The listing builds one solid part. Answer for the finished solid, in the listing's coordinates (mm). A direction names the side the tool comes from. Coordinates: 2 decimals unless noted, no trailing zeros. Write each loop counter-clockwise with the first axis right and the second up, starting at its lowest first coordinate (ties: lowest second). Pieces come first, ordered by that corner, then holes.
Autodesk Inventor part; units mm, degrees
ref_plane "YZ Plane" through (0, 0, 0) normal (1, 0, 0) x (0, 1, 0)
ref_plane "XZ Plane" through (0, 0, 0) normal (0, 1, 0) x (-1, 0, 0)
ref_plane "XY Plane" through (0, 0, 0) normal (0, 0, 1) x (1, 0, 0)
sketch "Esquisse1" plane through (0, 0, 0) normal (0, 0, 1) x (1, 0, 0)
  line L0 (0, 0) -> (-10, 0)
  line L1 (-10, 0) -> (-10, 30)
  line L2 (-10, 30) -> (0, 30)
  line L3 (0, 0) -> (-5, 0)
  line L4 (-5, 0) -> (-5, 5)
  line L5 (-5, 5) -> (0, 5)
  line L6 (0, 5) -> (0, 0)
  line L7 (0, 4) -> (-3, 4)
  line L8 (-3, 4) -> (-3, 1)
  line L9 (-3, 1) -> (0, 1)
  line L10 (0, 1) -> (0, 4)
  line L11 (-1.5, 5) -> (-1.5, 20)
  line L12 (-1.5, 20) -> (0, 20)
  line L13 (0, 30) -> (0, 20)
  line L14 (0, 5) -> (0, 0)
  line L15 (0, 29) -> (-3, 29)
  line L16 (-3, 29) -> (-3, 26)
  line L17 (-3, 26) -> (0, 26)
  line L18 (0, 26) -> (0, 29)
  line L19 (0, 25) -> (-5, 25)
  line L20 (-5, 25) -> (-5, 30)
  line L21 (-5, 25) -> (-7.5, 25)
  line L22 (-7.5, 25) -> (-7.5, 27.5)
  line L23 (-7.5, 27.5) -> (-5, 27.5)
  line L24 (-5, 27.5) -> (-5, 25)
  line L25 (-5, 0) -> (-7.5, 0)
  line L26 (-5, 2.5) -> (-5, 0)
  line L27 (-5, 5) -> (-7.5, 5)
  line L28 (-7.5, 5) -> (-7.5, 2.5)
  line L29 (-7.5, 2.5) -> (-5, 2.5)
  line L30 (-5, 2.5) -> (-5, 5)
  line L31 (-3, 26) -> (0, 26)
  line L32 (0, 26) -> (0, 29)
  line L33 (0, 29) -> (-3, 29)
  line L34 (-3, 29) -> (-3, 26)
  line L35 (-3, 1) -> (0, 1)
  line L36 (0, 1) -> (0, 4)
  line L37 (0, 4) -> (-3, 4)
  line L38 (-3, 4) -> (-3, 1)
  dimension "d0" = 10
  dimension "d1" = 30
  dimension "d2" = 5
  dimension "d3" = 5
  dimension "d4" = 3
  dimension "d5" = 3
  dimension "d6" = 1
  dimension "d7" = 15
  dimension "d9" = 3
  dimension "d10" = 3
  dimension "d11" = 1
  dimension "d12" = 5
  dimension "d13" = 5
  dimension "d14" = 2.5
  dimension "d15" = 2.5
  dimension "d20" = 2.5
  dimension "d21" = 2.5
extrude "Extrusion1" add sketch "Esquisse1" along normal blind 41.5 contours L0 L4 L5 L6 L7 L8 L9 | L9 L8 L7 L6 | L2 L13 L15 L16 L17 L19 L20 | L13 L17 L16 L15
extrude "Extrusion2" add sketch "Esquisse1" along normal blind 35 contours L29 L28 L27 L4 | L20 L21 L22 L23
extrude "Extrusion4" add sketch "Esquisse1" along normal blind 2 contours L0 L1 L2 L20 L23 L22 L21 L19 L13 L12 L11 L5 L27 L28 L29 L4
fillet "Congé1" radius 5 2 edges at (-10, 0, 1) (-10, 30, 1)
sketch "Esquisse3" plane through (0, 0, 0) normal (0, 0, -1) x (-1, 0, 0)
  circle A0 centre (7, 9) radius 0.7
  circle A1 centre (7, 21) radius 0.7
  line L0 (0, 0) -> (0, 5)
  line L1 (0, 20) -> (0, 30)
  line L2 (5, 0) -> (0, 0)
  dimension "d29" = 1.4
  dimension "d30" = 1.4
  dimension "d31" = 12
  dimension "d32" = 7
  dimension "d33" = 7
  dimension "d34" = 9
extrude "Extrusion5" cut sketch "Esquisse3" against normal through all
fillet "Congé2" radius 2 2 edges at (-3.75, 25, 2) (-4.5, 5, 2)
sketch "Esquisse8" plane through (0, 0, 41.5) normal (0, 0, 1) x (1, 0, 0)
  line L0 (0, 0) -> (0, 5)
  line L1 (0, 5) -> (-5, 5)
  line L2 (-5, 5) -> (-5, 0)
  line L3 (-5, 0) -> (0, 0)
  line L4 (0, 30) -> (-5, 30)
  line L5 (-5, 30) -> (-5, 25)
  line L6 (-5, 25) -> (0, 25)
  line L7 (0, 25) -> (0, 30)
  circle A0 centre (-2.5, 2.5) radius 2.4
  circle A1 centre (-2.5, 27.5) radius 2.4
  dimension "d42" = 4.8
  dimension "d43" = 2.5
  dimension "d44" = 2.5
  dimension "d45" = 4.8
  dimension "d48" = 2.5
  dimension "d49" = 2.5
extrude "Extrusion8" cut sketch "Esquisse8" against normal blind 6.5
sketch "Esquisse9" plane through (-2.5, 2.5, 41.5) normal (0, 0, 1) x (1, 0, 0)
  circle A0 centre (0, 0) radius 2.4
  circle A1 centre (0, 25) radius 2.4
  line L0 (0, 0) -> (3.9146, 0)
  circle A2 centre (1, 0) radius 1.4
  circle A3 centre (0, 0) radius 2.4
  line L1 (0, 25) -> (4.0517, 25)
  circle A4 centre (1, 25) radius 1.4
  point P0 (2.5, -2.5)
  dimension "d52" = 2.8
  dimension "d53" = 2.8
extrude "Extrusion9" cut sketch "Esquisse9" against normal blind 1.5
properties part number "blue_part-july21" material "Plastique ABS"
1. Section B-B on y = 9 is taken. Give the vertices of the cut face in (x, z).
Results found:
outline: (-10, 0) - (-7.7, 0) - (-7.7, 2) - (-10, 2) - close; (-6.3, 0) - (-1.5, 0) - (-1.5, 2) - (-6.3, 2) - close
2. For a pull along X with two mould halves and no side action, classify faces 1 (the cylindrical face through (-2.81, 4.88, 37.53)), 2 (the cylindrical face through (-6.909, 21.694, 0.986)), 3 (the flat face through (-3, 30, 17)) as pulls with the +X half, pulls with the -X half, needs draft (parallel to the pull), parting line crosses it, or undercut.
Results found:
face 1: parting line crosses it
face 2: undercut
face 3: needs draft
3. Section C-C on x = -1 is taken. Give the vertices of the cut face in (y, z), then the cut area to 3 significant figures.
Results found:
outline: (0, 0) - (5, 0) - (5, 35) - (4.37, 35) - (4.37, 40) - (3.81, 40) - (3.81, 41.5) - (1.19, 41.5) - (1.19, 40) - (0.63, 40) - (0.63, 35) - (0, 35) - close; (20, 0) - (30, 0) - (30, 35) - (29.37, 35) - (29.37, 40) - (28.81, 40) - (28.81, 41.5) - (26.19, 41.5) - (26.19, 40) - (25.63, 40) - (25.63, 35) - (25, 35) - (25, 4) arc R2 cw to (23, 2) - (20, 2) - close
area: 406 mm2
4. Flat-ended cylindrical pins translate along their axes: P1, Ø1.8, axis at x = -7, y = 9, coming from the +Z side; P2, Ø1.1, axis at x = -7, y = 21, coming from the -Z side; P3, Ø3.5, axis at y = 3.5, z = 18.5, coming from the -X side; P4, Ø3, axis at y = 12.5, z = 2, coming from the +X side. Find the tip coordinate at first contact, or state that the pin passes through.
Results found:
P1: stops at z = 2
P2: passes through
P3: stops at x = -7.5
P4: stops at x = -1.5
5. Find the intervals of material crossed by L1, parallel to Y at x = -7, z = 1.4; L2, parallel to Y at x = -6.5, z = 11; L3, parallel to Y at x = -3, z = 30, in increasing order.
Results found:
L1: y = 0.42 to 8.3, 9.7 to 20.3, 21.7 to 29.58
L2: y = 2.5 to 5, 25 to 27.5
L3: y = 0 to 5, 25 to 30
6. Section A-A on z = 17.5 is taken. Give the vertices of the cut face in (x, y), then the cut area to 3 significant figures.
Results found:
outline: (-7.5, 2.5) - (-5, 2.5) - (-5, 0) - (0, 0) - (0, 5) - (-7.5, 5) - close; (-7.5, 25) - (0, 25) - (0, 30) - (-5, 30) - (-5, 27.5) - (-7.5, 27.5) - close
area: 62.5 mm2
7. A tool of negligible diameter and unlimited length cuts with its end or side. For faces 4 (the cylindrical face through (-4.46, 5.57, 2.6)), 5 (the flat face through (-7.5, 26, 18)), 6 (the cylindrical face through (-1.803, 1.133, 40.76)), 7 (the flat face through (-6, 2.5, 18)), 8 (the flat face through (-5, 29, 18)), from which of +Z, -Z, +X, -X, +Y, -Y can it reach the whole face along a straight path? Write none if from no direction.
Results found:
face 4: +Z, +X, -X
face 5: +Z, -X, +Y, -Y
face 6: +Z
face 7: +Z, -X, -Y
face 8: +Z, -X, +Y
8. Section D-D on x = -7 is taken. Give the vertices of the cut face in (y, z).
Results found:
outline: (0.42, 0) - (8.3, 0) - (8.3, 2) - (7, 2) arc R2 cw to (5, 4) - (5, 35) - (2.5, 35) - (2.5, 2) - (0.42, 2) - close; (9.7, 0) - (20.3, 0) - (20.3, 2) - (9.7, 2) - close; (21.7, 0) - (29.58, 0) - (29.58, 2) - (27.5, 2) - (27.5, 35) - (25, 35) - (25, 4) arc R2 cw to (23, 2) - (21.7, 2) - close
